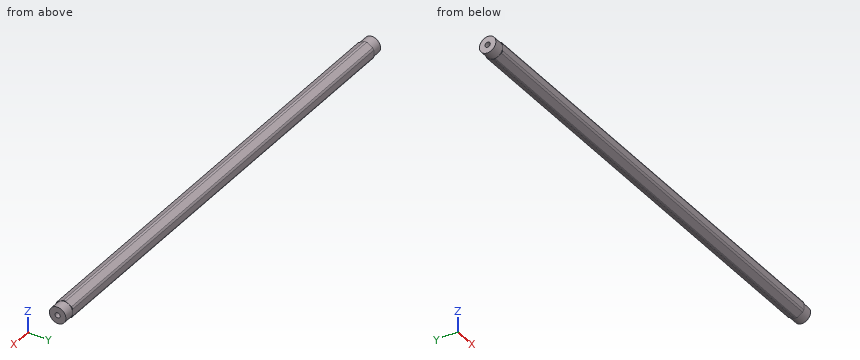
from build123d import *

# Parameters (mm, degrees)
SKETCH1_R               = 2.0193
BOSS_EXTRUDE1_DEPTH     = 184.15
SKETCH2_R               = 8.89
SKETCH2_R_2             = 6.35
CUT_EXTRUDE_THIN1_DEPTH = 7.9375


with BuildPart() as part:
    # Sketch1 → Boss-Extrude1 (new, symmetric)
    with BuildSketch(Plane(origin=(0, 0, 0), x_dir=(0, 0, -1), z_dir=(1, 0, 0))):
        with BuildLine():
            ThreePointArc((4.181770846, 5.456960429), (3.437499983, 5.953924622), (2.634980936, 6.35))
            Line((2.634980936, 6.35), (-2.634980936, 6.35))
            ThreePointArc((-2.634980936, 6.35), (-3.437499983, 5.953924622), (-4.181770846, 5.456960429))
            Line((-4.181770846, 5.456960429), (-6.816751782, 0.893039571))
            ThreePointArc((-6.816751782, 0.893039571), (-6.874999966, 0), (-6.816751782, -0.893039571))
            Line((-6.816751782, -0.893039571), (-4.181770846, -5.456960429))
            ThreePointArc((-4.181770846, -5.456960429), (-3.437499983, -5.953924622), (-2.634980936, -6.35))
            Line((-2.634980936, -6.35), (2.634980936, -6.35))
            ThreePointArc((2.634980936, -6.35), (3.437499983, -5.953924622), (4.181770846, -5.456960429))
            Line((4.181770846, -5.456960429), (6.816751782, -0.893039571))
            ThreePointArc((6.816751782, -0.893039571), (6.860422465, -0.447468582), (6.874999966, 0))
            ThreePointArc((6.874999966, 0), (6.860422465, 0.447468582), (6.816751782, 0.893039571))
            Line((6.816751782, 0.893039571), (4.181770846, 5.456960429))
        make_face()
        Circle(SKETCH1_R, mode=Mode.SUBTRACT)
    extrude(amount=BOSS_EXTRUDE1_DEPTH, both=True)

    # Sketch2 → Cut-Extrude-Thin1 (cut)
    with BuildSketch(Plane(origin=(184.15, 0, 0), x_dir=(0, 0, -1), z_dir=(1, 0, 0))):
        Circle(SKETCH2_R)
        Circle(SKETCH2_R_2, mode=Mode.SUBTRACT)
    cut_extrude_thin1 = extrude(amount=-CUT_EXTRUDE_THIN1_DEPTH, mode=Mode.SUBTRACT)

    # Mirror1: Cut-Extrude-Thin1 across plane
    add(cut_extrude_thin1.mirror(Plane(origin=(0, 0, 0), x_dir=(0, 0, 1), z_dir=(1, 0, 0))), mode=Mode.SUBTRACT)


solid = part.part
Build history of the part. All positions in model axes, mm. Round coordinates to 2 decimals unless told otherwise and drop trailing zeros. Write each loop counter-clockwise with the first axis right and the second up, starting at its lowest first coordinate (ties: lowest second). Pieces come first, ordered by that corner, then holes. Notation, with made-up numbers: (78, 29.5) -> (135, 29.5) arc R28 cw to (135, 50.5) -> close; hole circle Ø4 at (-19.5, 77). An arc over 180 degrees is marked (long way). Use one line per item in the form item = value.
Q1. Drill centre lines: L1, parallel to Y at x = -11.5, z = 0.5; L2, parallel to Z at x = 85.5, y = 0.25; L3, parallel to Y at x = -98, z = -2.75. Where is each one in solid material? Low to high.
Conclusion:
L1 = -6.35 to -1.96, 1.96 to 6.35
L2 = -6.87 to -2, 2 to 6.87
L3 = -6.3 to 6.3
Q2. Drop flat-ended pins along their axis: P1, Ø3, axis at x = -110.5, y = -2.5, coming from the -Z side (3 decimals); P2, Ø1, axis at x = 58, z = 3.5, coming from the +Y side; P3, Ø1, axis at x = -93.5, y = 1.5, coming from the +Z side (3 decimals). Give the stop position or say it passes through.
Conclusion:
P1 = -6.755
P2 = 6.19
P3 = 6.755
Q3. Band-saw the part on A-A, the plane x = 5.5. Write the cut outline in (y, z) (3 decimals).
Conclusion:
outline = (-6.35, -2.635) arc R6.875 ccw to (-5.457, -4.182) -> (-0.893, -6.817) arc R6.875 ccw to (0.893, -6.817) -> (5.457, -4.182) arc R6.875 ccw to (6.35, -2.635) -> (6.35, 2.635) arc R6.875 ccw to (5.457, 4.182) -> (0.893, 6.817) arc R6.875 ccw to (-0.893, 6.817) -> (-5.457, 4.182) arc R6.875 ccw to (-6.35, 2.635) -> close; hole circle Ø4.039 at (0, 0)
